Read the model definition and answer for the solid it produces. Units are mm, in the model's axes. Face numbers are marked on the shaded views. A direction names the side the tool comes from. Round coordinates to 2 decimals unless told otherwise and drop trailing zeros. Loops run counter-clockwise (first coordinate to the right, second up) from the corner with the lowest first, then second, coordinate; pieces in that order, holes last. Notation, with made-up numbers: (56.25, 69) - (94.25, 69) arc R16 ccw to (94.25, 73) - close; hole circle Ø4 at (15.5, 81). An arc over 180 degrees is marked (long way). Use CSV: the item, a comma, the result in double quotes. Start each with the question number.
1. Consider line 1 along X through (y, z) = (20.75, -8); line 2 along X through (y, z) = (12.25, 2.5); line 3 along Y through (x, z) = (29, 14). Determine where each line is inside the solid, lowest interval first.
2. Find section D-D (z = 14). State how many separate pieces and enclosed holes the cut face has, and give its area (3 significant figures).
3. Find section B-B (x = 53). Give the vertices of the cut face in (y, z), and give its area (3 significant figures).
4. A tool of negligible diameter and unlimited length cuts with its end or side. For the marked faces 1, 2 and 3, from which of +Z, -Z, +X, -X, +Y, -Y can it reach the whole face along a straight path? Write none if from no direction.
5. Given pin 1 Ø11 at (x, z) = (48.5, -12) entering from +Y; pin 2 Ø3 at (x, y) = (40, 20) entering from +Z; pin 3 Ø4.5 at (y, z) = (13, -10) entering from -X, each flat-ended and moving along its own axis, determine where each tip first touches the part or whether it passes through.
6. Find section C-C (y = 5.25). Give the vertices of the cut face in (x, z).
7. Determine the mould class of the marked faces 4, 5, 6 and 7 for opening direction Y: +Y half, -Y half, draft (parallel to the pull), parting line (faces both ways), or undercut.
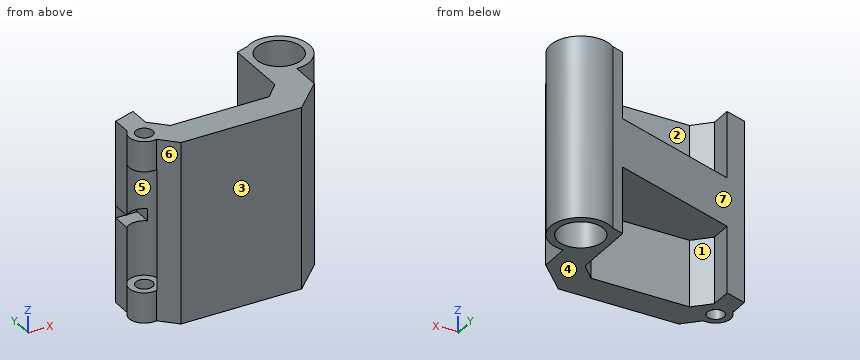
from build123d import *

# Parameters (mm, degrees)
BOSS_EXTRUDE1_DEPTH             = 19.05
BOSS_EXTRUDE1_DEPTH_BACK        = 19.05
SKETCH5_R                       = 6.35
BOSS_EXTRUDE2_DEPTH             = 38.1
F_3_8_0_375_DIAMETER_HOLE1_D    = 9.525
CUT_EXTRUDE2_DEPTH              = 38.1
CUT_EXTRUDE5_DEPTH              = 13.97
CUT_EXTRUDE6_DEPTH              = 13.97
CUT_EXTRUDE7_DEPTH              = 39.1
BOSS_EXTRUDE5_DEPTH             = 38.1
BOSS_EXTRUDE6_DEPTH             = 38.1
F_9_64_0_14063_DIAMETER_HOLE2_D = 3.572002
SKETCH25_R                      = 3.302
CUT_EXTRUDE8_DEPTH              = 12.7
CUT_EXTRUDE8_DEPTH_BACK         = 12.7
SKETCH28_W                      = 2.54
SKETCH28_H                      = 4.012120109
CUT_EXTRUDE9_DEPTH              = 4.499728


with BuildPart() as part:
    # Sketch4 → Boss-Extrude1 (new body, two sides)
    with BuildSketch(Plane.XY) as boss_extrude1_sk:
        Polygon((25.4, 1.404612262), (25.4, 14.104612262), (63.5, 26.804612262), (63.5, 1.404612262), align=None)
    extrude(amount=BOSS_EXTRUDE1_DEPTH)
    extrude(boss_extrude1_sk.sketch, amount=-BOSS_EXTRUDE1_DEPTH_BACK)

    # Sketch5 → Boss-Extrude2 (add)
    with BuildSketch(Plane.XY.offset(19.05)):
        with Locations((63.5, 20.454612262)):
            Circle(SKETCH5_R)
    extrude(amount=-BOSS_EXTRUDE2_DEPTH)

    # 3/8 (0.375) Diameter Hole1 (through all)
    with Locations(Plane.XY.offset(19.05)):
        with Locations((63.5, 20.454612262)):
            Hole(F_3_8_0_375_DIAMETER_HOLE1_D / 2)

    # Sketch11 → Cut-Extrude2 (cut)
    with BuildSketch(Plane.XY.offset(19.05)):
        Polygon((63.5, 7.754612262), (57.15, 1.404612262), (63.5, 1.404612262), align=None)
    extrude(amount=-CUT_EXTRUDE2_DEPTH, mode=Mode.SUBTRACT)

    # Sketch20 → Cut-Extrude5 (cut)
    with BuildSketch(Plane.XY.offset(19.05)):
        Polygon((29.899727951, 7.754612262), (53.975, 7.754612262), (57.15, 11.056612262), (57.15, 24.687945595), (29.899727951, 15.604521579), align=None)
    extrude(amount=-CUT_EXTRUDE5_DEPTH, mode=Mode.SUBTRACT)

    # Sketch21 → Cut-Extrude6 (cut)
    with BuildSketch(Plane(origin=(0, 0, -19.05), x_dir=(-1, 0, 0), z_dir=(0, 0, -1))):
        Polygon((-57.15, 24.687945595), (-57.15, 11.056612262), (-53.975, 7.754612262), (-29.899727951, 7.754612262), (-29.899727951, 15.604521579), align=None)
    extrude(amount=-CUT_EXTRUDE6_DEPTH, mode=Mode.SUBTRACT)

    # Sketch11<4> → Cut-Extrude7 (cut, through all)
    with BuildSketch(Plane.XY.offset(19.05)):
        Polygon((25.4, 7.754612262), (31.75, 1.404612262), (25.4, 1.404612262), align=None)
    extrude(amount=-CUT_EXTRUDE7_DEPTH, mode=Mode.SUBTRACT)

    # Sketch22 → Boss-Extrude5 (add)
    with BuildSketch(Plane.XY.offset(19.05)):
        Polygon((33.201727951, 7.754612262), (29.899727951, 11.056612262), (29.899727951, 7.754612262), align=None)
    extrude(amount=-BOSS_EXTRUDE5_DEPTH)

    # Sketch23 → Boss-Extrude6 (add)
    with BuildSketch(Plane.XY.offset(19.05)):
        with BuildLine():
            ThreePointArc((28.484500237, 4.670112024), (30.228876772, 5.793622896), (30.906849398, 7.754612262))
            ThreePointArc((30.906849398, 7.754612262), (28.888785689, 10.711320469), (25.4, 9.909398419))
            Line((25.4, 9.909398419), (25.4, 7.754612262))
            Line((25.4, 7.754612262), (28.484500237, 4.670112024))
        make_face()
        with BuildLine():
            Line((25.4, 7.754612262), (25.4, 9.909398419))
            ThreePointArc((25.4, 9.909398419), (24.9957943, 6.143827516), (28.484500237, 4.670112024))
            Line((28.484500237, 4.670112024), (25.4, 7.754612262))
        make_face()
    extrude(amount=-BOSS_EXTRUDE6_DEPTH)

    # 9/64 (0.14063) Diameter Hole2 (through all)
    with Locations(Plane(origin=(27.731849398, 7.754612262, 19.05), x_dir=(1, 0, 0), z_dir=(0, 0, 1))):
        with Locations((0, 0)):
            Hole(F_9_64_0_14063_DIAMETER_HOLE2_D / 2)

    # Sketch25 → Cut-Extrude8 (cut, two sides)
    with BuildSketch(Plane.XY) as cut_extrude8_sk:
        with Locations((27.731849398, 7.754612262)):
            Circle(SKETCH25_R)
    extrude(amount=CUT_EXTRUDE8_DEPTH, mode=Mode.SUBTRACT)
    extrude(cut_extrude8_sk.sketch, amount=-CUT_EXTRUDE8_DEPTH_BACK, mode=Mode.SUBTRACT)

    # Sketch28 → Cut-Extrude9 (cut)
    with BuildSketch(Plane.ZY.offset(-25.4)):
        with Locations((0, 12.098552208)):
            Rectangle(SKETCH28_W, SKETCH28_H)
    extrude(amount=-CUT_EXTRUDE9_DEPTH, mode=Mode.SUBTRACT)


solid = part.part
Filled sheet:
1,line 1,"x = 57.15 to 58.75, 68.25 to 69.84"
1,line 2,"x = 25.4 to 63.5"
1,line 3,"y = 4.15 to 6.5, 9.01 to 15.3"
2,separate pieces,"1"
2,enclosed holes,"2"
2,area,"348 mm²"
3,outline,"(1.4, -19.05) - (7.75, -19.05) - (7.75, -5.08) - (23.3, -5.08) - (23.3, 5.08) - (7.75, 5.08) - (7.75, 19.05) - (1.4, 19.05) - close"
3,area,"400 mm²"
4,face 1,"-Z, +Y"
4,face 2,"+Z, +Y"
4,face 3,"+Z, -Z, +X, -X, -Y"
5,pin 1,"stops at y = 7.78"
5,pin 2,"stops at z = 5.08"
5,pin 3,"stops at x = 25.4"
6,outline,"(25.78, -19.05) - (61, -19.05) - (61, 19.05) - (25.78, 19.05) - (25.78, 12.7) - (29.88, 12.7) - (29.88, -12.7) - (25.78, -12.7) - close"
7,face 4,"draft"
7,face 5,"undercut"
7,face 6,"-Y half"
7,face 7,"+Y half"
